```python
from build123d import *

# Parameters (mm, degrees)
SKETCH1_W           = 6
SKETCH1_H           = 5
BOSS_EXTRUDE1_DEPTH = 6
CUT_EXTRUDE1_DEPTH  = 2.5


with BuildPart() as part:
    # Sketch1 → Boss-Extrude1 (new body)
    with BuildSketch(Plane(origin=(0, 0, 0), x_dir=(1, 0, 0), z_dir=(0, 1, 0))):
        Rectangle(SKETCH1_W, SKETCH1_H)
    extrude(amount=BOSS_EXTRUDE1_DEPTH)

    # Sketch2 → Cut-Extrude1 (cut)
    with BuildSketch(Plane(origin=(0, 6, 0), x_dir=(1, 0, 0), z_dir=(0, 1, 0))):
        Polygon((3, -1), (0, -1), (0, 1), (-3, 1), (-3, -2.5), (3, -2.5), align=None)
    extrude(amount=-CUT_EXTRUDE1_DEPTH, mode=Mode.SUBTRACT)


solid = part.part
```
Model file for the job. Use its own axes, mm. A direction names the side the tool comes from. Coordinates: 2 decimals unless noted, no trailing zeros. Loops run counter-clockwise (first coordinate to the right, second up) from the corner with the lowest first, then second, coordinate; pieces in that order, holes last. Notation, with made-up numbers: (61, -27.5) -> (90, -27.5) arc R8 ccw to (90, -23.5) -> close; hole circle Ø8 at (-38, 37). An arc over 180 degrees is marked (long way). Answer as a JSON object with one key per item and string values.
Q1. Cut at C-C (z = 1.9). List the corners of the cut face in (x, y).
Report:
{"outline": "(-3, 0) -> (3, 0) -> (3, 3.5) -> (-3, 3.5) -> close"}
Q2. 3-axis set-ups, long thin cutter, end or side, ignore diameter. For faces 1 (the flat face through (0, 0, 0)), 2 (the flat face through (2, 5, 1)), 3 (the flat face through (-1, 5, -1)): which of +Z, -Z, +X, -X, +Y, -Y reach the whole face in a straight line?
Report:
{"face 1": "+Z, -Z, +X, -X, -Y", "face 2": "+Z, +X, -X, +Y", "face 3": "+Z, -X, +Y"}
Q3. Probe probe 1 along Y at (x, z) = (1.25, 2.15); probe 2 along X at (y, z) = (5.5, 0.4); probe 3 along Z at (x, y) = (2.55, 5.05). List the from-to ranges inside material, lowest first.
Report:
{"probe 1": "y = 0 to 3.5", "probe 2": "x = 0 to 3", "probe 3": "z = -2.5 to 1"}
Q4. Cut at B-B (z = -0.1). List the corners of the cut face in (x, y), and give its area (3 significant figures).
Report:
{"outline": "(-3, 0) -> (3, 0) -> (3, 6) -> (0, 6) -> (0, 3.5) -> (-3, 3.5) -> close", "area": "28.5 mm2"}
Q5. Cut at A-A (x = 0.4). List the corners of the cut face in (y, z).
Report:
{"outline": "(0, -2.5) -> (6, -2.5) -> (6, 1) -> (3.5, 1) -> (3.5, 2.5) -> (0, 2.5) -> close"}
Q6. Flat gauge pin, fed straight in: P1, Ø1.2, axis at x = 2, y = 4, coming from the +Z side. Where does the tip first touch, or does it go through?
Report:
{"P1": "stops at z = 2.5"}
